The drawing under review shows one solid part. Ordinate dimensions are in mm from its lowest x, y, z. A direction names the side the tool comes from. Round coordinates to 2 decimals unless told otherwise and drop trailing zeros. Order: outer loops, then holes, each group sorted by start corner. A loop starts at its lowest first (then second) coordinate and runs counter-clockwise, first axis right, second up. Notation, with made-up numbers: (-6.75, 82) -> (6.25, 82) arc R16 cw to (6.25, 96) -> close; hole circle Ø5 at (69.5, 26.25). An arc over 180 degrees is marked (long way). Return JSON: item names as keys, results as strings. Group by question number.
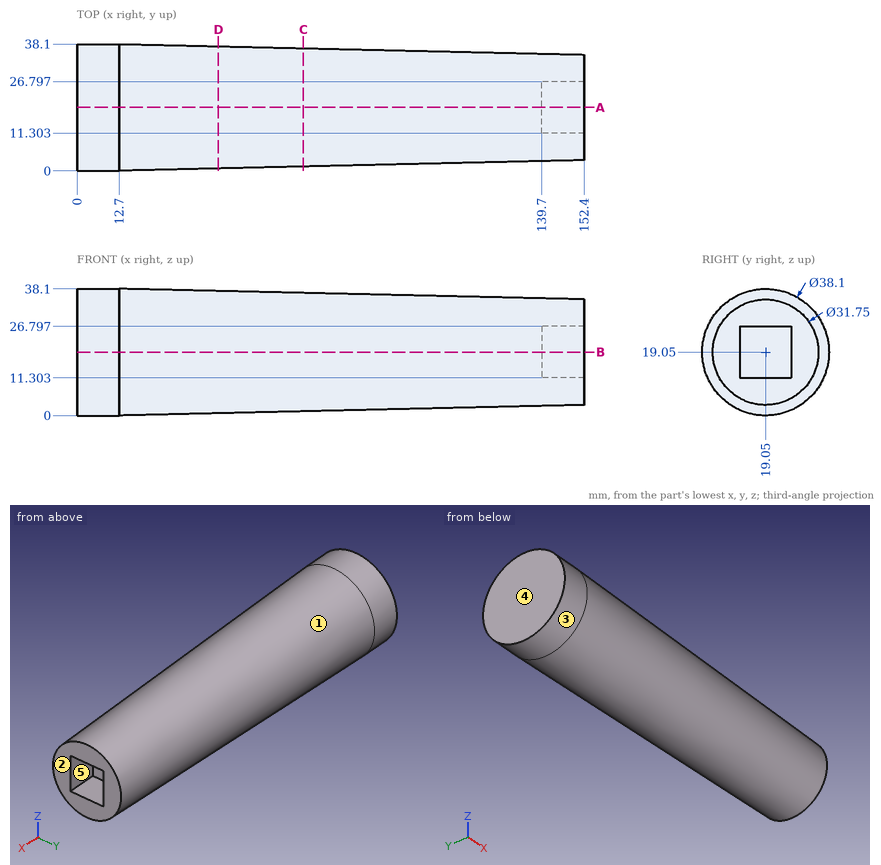
Item 1: Consider section A-A on y = 19.05. State the section outline as (x, z) points (3 decimals).
Item 2: For the marked faces 1 and 2, list the 3-axis set-ups (+Z, -Z, +X, -X, +Y, -Y) from which the entire face can be reached by the end or side of a thin tool; tool diameter is ignored.
Item 3: The part is to be moulded in two halves that separate along Y. For the marked faces 3, 4 and 5, say which applies: +Y half, -Y half, draft (parallel to the pull), parting line (faces both ways), or undercut.
Item 4: Insertion check: pin 1 Ø10 at (x, y) = (80.5, 33.5) entering from -Z; pin 2 Ø8 at (x, z) = (44, 22.5) entering from -Y; pin 3 Ø12 at (x, y) = (49.5, 29) entering from +Z. Each pin has a flat end and moves straight along its axis. Give the tip position at first contact, or say it passes through.
Item 5: Consider section C-C on x = 68. State the section outline as (y, z) points.
Item 6: Wall thickness on line 1 along X through (y, z) = (25.5, 12.5); line 2 along Z through (x, y) = (144, 24); line 3 along Z through (x, y) = (69, 27): over which ranges is each line inside the solid? List them lowest first.
Item 7: Consider section D-D on x = 42.5. State the section outline as (y, z) points.
Values:
{
 "1": {"outline": "(0, 0) -> (12.7, 0) -> (152.4, 3.175) -> (152.4, 11.303) -> (139.7, 11.303) -> (139.7, 26.797) -> (152.4, 26.797) -> (152.4, 34.925) -> (12.7, 38.1) -> (0, 38.1) -> close"},
 "2": {"face 1": "+X", "face 2": "+Z, -Z, +X, +Y, -Y"},
 "3": {"face 3": "parting line", "face 4": "draft", "face 5": "undercut"},
 "4": {"pin 1": "z = 4.31", "pin 2": "y = 0.66", "pin 3": "z = 36.84"},
 "5": {"outline": "circle Ø35.59 at (19.05, 19.05)"},
 "6": {"line 1": "0 to 139.7", "line 2": "3.77 to 11.3, 26.8 to 34.33", "line 3": "3.16 to 34.94"},
 "7": {"outline": "circle Ø36.75 at (19.05, 19.05)"}
}
